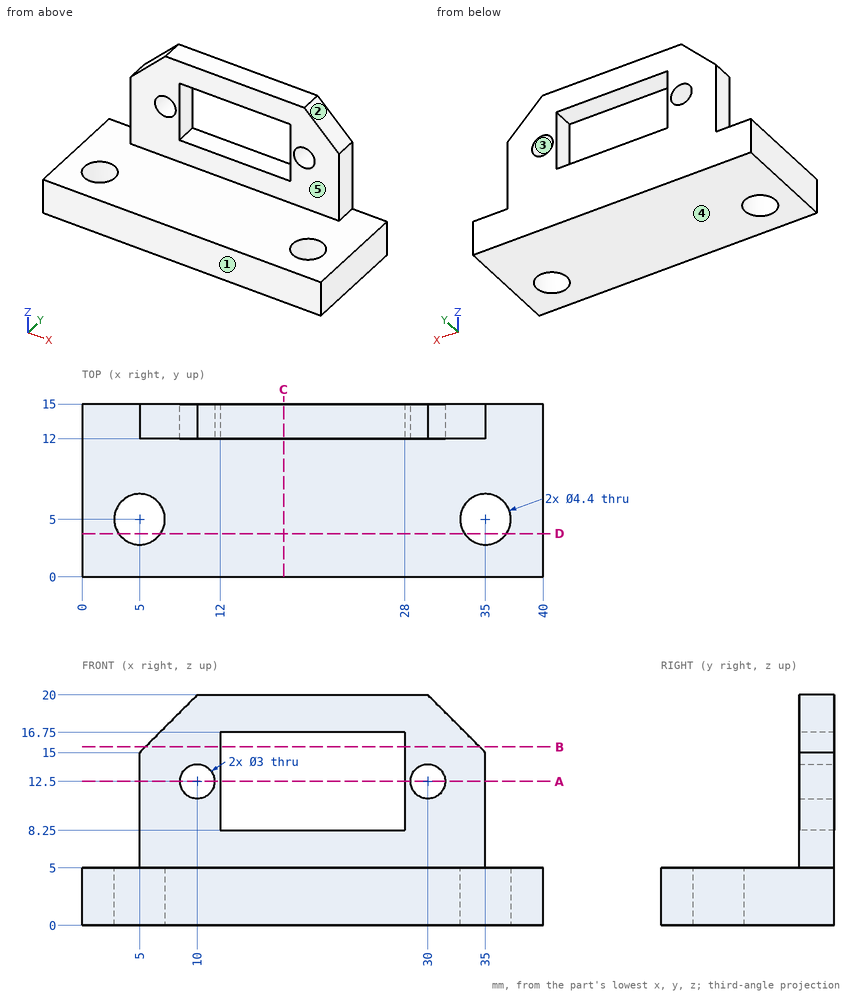
Source: three-view drawing plus pictorial views. Frame: mm from the lowest corner of the part. A direction names the side the tool comes from. Give positions to 0.01 mm unless a question says otherwise; leave off trailing zeros. Order: outer loops, then holes, each group sorted by start corner. A loop starts at its lowest first (then second) coordinate and runs counter-clockwise, first axis right, second up. Notation, with made-up numbers: M 79,40 L 106,40 A20 cw 106,78 Z; hole C -9,15 d7. An arc over 180 degrees is marked long. One line per question, with ' | ' between items.
1) Contact query for flat-ended pins moving along their axis: P1, Ø3.5, axis at y = 13, z = 12.5, coming from the +X side; P2, Ø2.5, axis at y = 14, z = 14.5, coming from the -X side; P3, Ø3, axis at x = 27.5, z = 12.5, coming from the -Y side. Output: stop coordinate, or through.
Filled in:
P1: stops at x = 35 | P2: stops at x = 5 | P3: stops at y = 12
2) Section B-B on z = 15.5. Output: boundary loops of the cut face in (x, y), and give its area (3 significant figures).
Filled in:
outline: M 5.5,12 L 12,12 L 12,15 L 5.5,15 Z; M 28,12 L 34.5,12 L 34.5,15 L 28,15 Z | area: 39.0 mm2
3) Ray query, L1, parallel to X at y = 14.1, z = 12.5; L2, parallel to Y at x = 35, z = 2.2; L3, parallel to Z at x = 26.5, y = 12.25. Return the intervals inside material, ascending.
Filled in:
L1: x = 5 to 8.5, 11.5 to 12, 28 to 28.5, 31.5 to 35 | L2: y = 0 to 2.8, 7.2 to 15 | L3: z = 0 to 8.25, 16.75 to 20
4) Draft query along Z for the marked faces 1, 2 and 3. Return one class per face: pulls with the +Z half, pulls with the -Z half, needs draft (parallel to the pull), parting line crosses it, or undercut.
Filled in:
face 1: needs draft | face 2: pulls with the +Z half | face 3: undercut
5) Access query for the marked faces 4 and 5. Directions: +Z, -Z, +X, -X, +Y, -Y. A direction counts if a zero-diameter tool reaches every point of the face in a straight line with its end or side. Return the directions, or none.
Filled in:
face 4: -Z, +X, -X, +Y, -Y | face 5: +Z, +X, -X, -Y
6) Section C-C on x = 17.5. Output: boundary loops of the cut face in (y, z), and give its area (3 significant figures).
Filled in:
outline: M 0,0 L 15,0 L 15,8.25 L 12,8.25 L 12,5 L 0,5 Z; M 12,16.75 L 15,16.75 L 15,20 L 12,20 Z | area: 94.5 mm2
7) Section D-D on y = 3.75. Output: boundary loops of the cut face in (x, z), and give its area (3 significant figures).
Filled in:
outline: M 0,0 L 3.19,0 L 3.19,5 L 0,5 Z; M 6.81,0 L 33.19,0 L 33.19,5 L 6.81,5 Z; M 36.81,0 L 40,0 L 40,5 L 36.81,5 Z | area: 164 mm2
8) Section A-A on z = 12.5. Output: boundary loops of the cut face in (x, y).
Filled in:
outline: M 5,12 L 8.5,12 L 8.5,15 L 5,15 Z; M 11.5,12 L 12,12 L 12,15 L 11.5,15 Z; M 28,12 L 28.5,12 L 28.5,15 L 28,15 Z; M 31.5,12 L 35,12 L 35,15 L 31.5,15 Z
